from build123d import *

# Parameters (mm, degrees)
CROQUIS1_W              = 40.5
CROQUIS1_H              = 20.2
SALIENTE_EXTRUIR1_DEPTH = 36.8
CROQUIS2_R              = 9.710333118
SALIENTE_EXTRUIR2_DEPTH = 2.44
CROQUIS3_R              = 2.5
SALIENTE_EXTRUIR3_DEPTH = 5.66
CROQUIS4_W              = 20.2
CROQUIS4_H              = 2.5
SALIENTE_EXTRUIR4_DEPTH = 6.88
CROQUIS5_W              = 20.2
CROQUIS5_H              = 2.5
SALIENTE_EXTRUIR5_DEPTH = 6.88
CORTAR_EXTRUIR1_DEPTH   = 32.3


with BuildPart() as part:
    # Croquis1 → Saliente-Extruir1 (new body)
    with BuildSketch(Plane(origin=(0, 0, 0), x_dir=(1, 0, 0), z_dir=(0, 1, 0))):
        with Locations((20.25, 10.1)):
            Rectangle(CROQUIS1_W, CROQUIS1_H)
    extrude(amount=SALIENTE_EXTRUIR1_DEPTH)

    # Croquis2 → Saliente-Extruir2 (add)
    with BuildSketch(Plane(origin=(0, 36.8, 0), x_dir=(1, 0, 0), z_dir=(0, 1, 0))):
        with Locations((25.5, 10.1)):
            Circle(CROQUIS2_R)
        with BuildLine():
            Line((18.770173162, 17.1), (8.106469176, 17.1))
            Line((8.106469176, 17.1), (8.106469176, 3.1))
            Line((8.106469176, 3.1), (18.770173162, 3.1))
            ThreePointArc((18.770173162, 3.1), (15.789666882, 10.1), (18.770173162, 17.1))
        make_face()
    extrude(amount=SALIENTE_EXTRUIR2_DEPTH)

    # Croquis3 → Saliente-Extruir3 (add)
    with BuildSketch(Plane(origin=(0, 39.24, 0), x_dir=(1, 0, 0), z_dir=(0, 1, 0))):
        with Locations((25.5, 10.1)):
            Circle(CROQUIS3_R)
    extrude(amount=SALIENTE_EXTRUIR3_DEPTH)

    # Croquis4 → Saliente-Extruir4 (add)
    with BuildSketch(Plane.ZY):
        with Locations((-10.1, 30.05)):
            Rectangle(CROQUIS4_W, CROQUIS4_H)
    extrude(amount=SALIENTE_EXTRUIR4_DEPTH)

    # Croquis5 → Saliente-Extruir5 (add)
    with BuildSketch(Plane(origin=(40.5, 0, 0), x_dir=(0, 0, -1), z_dir=(1, 0, 0))):
        with Locations((10.1, 30.05)):
            Rectangle(CROQUIS5_W, CROQUIS5_H)
    extrude(amount=SALIENTE_EXTRUIR5_DEPTH)

    # Croquis6 → Cortar-Extruir1 (cut, through all)
    with BuildSketch(Plane(origin=(0, 31.3, 0), x_dir=(1, 0, 0), z_dir=(0, 1, 0))):
        with BuildLine():
            ThreePointArc((-6.88, 4.717651116), (-3, 5.4), (-6.88, 6.082348884))
            Line((-6.88, 6.082348884), (-6.88, 4.717651116))
        make_face()
        with BuildLine():
            ThreePointArc((-6.88, 14.117651116), (-3, 14.8), (-6.88, 15.482348884))
            Line((-6.88, 15.482348884), (-6.88, 14.117651116))
        make_face()
        with BuildLine():
            Line((47.38, 14.117651116), (47.38, 15.482348884))
            ThreePointArc((47.38, 15.482348884), (43.5, 14.8), (47.38, 14.117651116))
        make_face()
        with BuildLine():
            Line((47.38, 4.717651116), (47.38, 6.082348884))
            ThreePointArc((47.38, 6.082348884), (43.5, 5.4), (47.38, 4.717651116))
        make_face()
    extrude(amount=-CORTAR_EXTRUIR1_DEPTH, mode=Mode.SUBTRACT)


solid = part.part
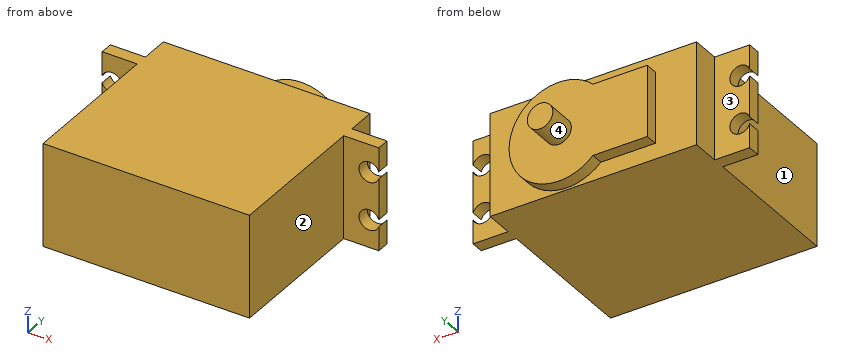
Could you check a few things on this model? Use its own coordinates, in mm. Face numbers are marked on the shaded views. A direction names the side the tool comes from. Give positions to 0.01 mm unless a question says otherwise; leave off trailing zeros. Order: outer loops, then holes, each group sorted by start corner. A loop starts at its lowest first (then second) coordinate and runs counter-clockwise, first axis right, second up.
1. Suppose I cut it at A-A (x = 45.5). List the corners of the cut face in (y, z) for me, plus the area to 3 significant figures.
2. Suppose I cut it at C-C (z = -11.75). List the corners of the cut face in (x, y) for me.
3. Suppose I cut it at B-B (x = 13.5). List the corners of the cut face in (y, z) for me, plus the area to 3 significant figures.
4. I need wall thicknesses on L1, parallel to Z at x = -5, y = 30.15; L2, parallel to Y at x = 33, z = -10; L3, parallel to X at y = 5, z = -16.25. Which ranges of each line are inside material? Lowest first, please.
5. For the marked faces 1, 2, 3 and 4, which set-ups out of +Z, -Z, +X, -X, +Y, -Y let a thin tool reach every point of the face, with its end or its side?
6. Will these pins go through, and if not, where does the flat tip stop? P1, Ø12, axis at x = 18.5, z = -4, coming from the +Y side; P2, Ø2, axis at x = 43, z = -6, coming from the -Y side; P3, Ø8, axis at x = 4.5, z = -15.5, coming from the -Y side; P4, Ø1.6, axis at y = 33.5, z = -13, coming from the +X side.
7. Suppose I cut it at D-D (x = 25.5). List the corners of the cut face in (y, z) for me, plus the area to 3 significant figures.
Solved:
1. outline: (28.8, -20.2) - (31.3, -20.2) - (31.3, -16.8) - (28.8, -16.8) - close; (28.8, -12.8) - (31.3, -12.8) - (31.3, -7.4) - (28.8, -7.4) - close; (28.8, -3.4) - (31.3, -3.4) - (31.3, 0) - (28.8, 0) - close
1. area: 30.5 mm2
2. outline: (-6.88, 28.8) - (0, 28.8) - (0, 0) - (40.5, 0) - (40.5, 28.8) - (47.38, 28.8) - (47.38, 31.3) - (40.5, 31.3) - (40.5, 36.8) - (35.07, 36.8) - (35.07, 39.24) - (27.38, 39.24) - (27.38, 44.9) - (23.62, 44.9) - (23.62, 39.24) - (8.11, 39.24) - (8.11, 36.8) - (0, 36.8) - (0, 31.3) - (-6.88, 31.3) - close
3. outline: (0, -20.2) - (36.8, -20.2) - (36.8, -17.1) - (39.24, -17.1) - (39.24, -3.1) - (36.8, -3.1) - (36.8, 0) - (0, 0) - close
3. area: 778 mm2
4. L1: z = -20.2 to -16.8, -12.8 to -7.4, -3.4 to 0
4. L2: y = 0 to 39.24
4. L3: x = 0 to 40.5
5. face 1: +Z, -Z, -X, -Y
5. face 2: +Z, -Z, +X, -Y
5. face 3: +Z, -Z, -X, +Y
5. face 4: +Y
6. P1: stops at y = 39.24
6. P2: stops at y = 28.8
6. P3: stops at y = 0
6. P4: stops at x = 40.5
7. outline: (0, -20.2) - (36.8, -20.2) - (36.8, -19.81) - (39.24, -19.81) - (39.24, -12.6) - (44.9, -12.6) - (44.9, -7.6) - (39.24, -7.6) - (39.24, -0.39) - (36.8, -0.39) - (36.8, 0) - (0, 0) - close
7. area: 819 mm2
